Read the model definition and answer for the solid it produces. Units are mm, in the model's axes. A direction names the side the tool comes from. Give positions to 0.01 mm unless a question says otherwise; leave off trailing zeros. Write each loop counter-clockwise with the first axis right and the second up, starting at its lowest first coordinate (ties: lowest second). Pieces come first, ordered by that corner, then holes. Notation, with made-up numbers: (-19.75, 87.25) -> (31.25, 87.25) arc R15 cw to (31.25, 101.25) -> close; hole circle Ø6 at (13.5, 74). An arc over 180 degrees is marked (long way). Write item = value, one per line.
Autodesk Fusion 360 part; units mm, degrees
sketch "Sketch1" plane through (0, 0, 0) normal (0, 0, 1) x (1, 0, 0)
  line L0 (0, 0) -> (51, 0)
  line L1 (51, 0) -> (51, 144)
  line L2 (51, 144) -> (0, 144)
  line L3 (0, 144) -> (0, 0)
  line L4 (10, 10) -> (41, 10)
  line L5 (41, 10) -> (41, 134)
  line L6 (41, 134) -> (10, 134)
  line L7 (10, 134) -> (10, 10)
  dimension "d1" = 51
  dimension "d2" = 144
  dimension "d5" = 31
  dimension "d6" = 124
extrude "Extrude1" add sketch "Sketch1" along normal blind 13
sketch "Sketch2" plane through (0, 0, 0) normal (0, 0, -1) x (1, 0, 0)
  line L0 (10, -134) -> (10, -10)
  line L1 (10, -10) -> (41, -10)
  line L2 (41, -10) -> (41, -134)
  line L3 (41, -134) -> (10, -134)
  line L4 (0, 0) -> (0, -144)
  line L5 (0, -144) -> (51, -144)
  line L6 (51, -144) -> (51, 0)
  line L7 (51, 0) -> (0, 0)
  line L8 (41, -134) -> (10, -134)
  line L9 (10, -134) -> (10, -10)
  line L10 (10, -10) -> (41, -10)
  line L11 (41, -10) -> (41, -134)
extrude "Extrude2" add sketch "Sketch2" against normal blind 3 contours L0 L1 L2 L3 L8 L9 L10 L11
sketch "Sketch3" plane through (0, 0, 13) normal (0, 0, 1) x (-1, 0, 0)
  line L0 (-10, -10) -> (-10, -134)
  line L1 (-10, -134) -> (-41, -134)
  line L2 (-41, -134) -> (-41, -10)
  line L3 (-41, -10) -> (-10, -10)
  line L4 (0, -144) -> (0, 0)
  line L5 (0, 0) -> (-51, 0)
  line L6 (-51, 0) -> (-51, -144)
  line L7 (-51, -144) -> (0, -144)
  line L8 (-41, -48.7) -> (-41, -67.4)
  line L9 (-41, -48.7) -> (-51, -48.7)
  line L10 (-51, -48.7) -> (-51, -67.4)
  line L11 (-51, -67.4) -> (-41, -67.4)
  line L12 (-41, -67.4) -> (-41, -48.7)
  dimension "d11" = 38.7
  dimension "d12" = 18.7
  dimension "d13" = 18.7
extrude "Extrude3" cut sketch "Sketch3" against normal blind 10 contours L2 L6 L8 L9 L10 L11 L12
(1) The part is cut by section B-B on y = 47. Determine the outline of the cut face in (x, z).
Checks:
outline = (0, 0) -> (51, 0) -> (51, 13) -> (41, 13) -> (41, 3) -> (10, 3) -> (10, 13) -> (0, 13) -> close
(2) The part is cut by section A-A on x = 16. Determine the outline of the cut face in (y, z), plus the area to 3 significant figures.
Checks:
outline = (0, 0) -> (144, 0) -> (144, 13) -> (134, 13) -> (134, 3) -> (10, 3) -> (10, 13) -> (0, 13) -> close
area = 632 mm²
(3) Given P1, Ø5, axis at x = 45.5, z = 3.5, coming from the -Y side, flat-ended and moving along its own axis, determine where the tip first touches the part or whether it passes through.
Checks:
P1 = 0
(4) For a pull along X with two mould halves and no side action, classify faces 1 (the flat face through (26, 134, 8)), 2 (the flat face through (51, 71, 6)), 3 (the flat face through (46, 67.4, 8)) as released by +X, released by -X, zero draft, split by the parting line, or undercut.
Checks:
face_1 = undercut
face_2 = released by +X
face_3 = zero draft
(5) Consider L1, parallel to X at y = 15, z = 12.25; L2, parallel to Y at x = 38, z = 6.5; L3, parallel to Y at x = 43, z = 10.5. Determine where each line is inside the solid, lowest interval first.
Checks:
L1 = 0 to 10, 41 to 51
L2 = 0 to 10, 134 to 144
L3 = 0 to 48.7, 67.4 to 144
(6) A tool of negligible diameter and unlimited length cuts with its end or side. For faces 4 (the flat face through (8, 73, 13)), 5 (the flat face through (10, 73, 8)), 6 (the flat face through (46, 48.7, 8)), from which of +Z, -Z, +X, -X, +Y, -Y can it reach the whole face along a straight path? Write none if from no direction.
Checks:
face_4 = +Z, +X, -X, +Y, -Y
face_5 = +Z
face_6 = +Z, +X
(7) The part is cut by section C-C on z = 7. Determine the outline of the cut face in (x, y), plus the area to 3 significant figures.
Checks:
outline = (0, 0) -> (51, 0) -> (51, 48.7) -> (41, 48.7) -> (41, 10) -> (10, 10) -> (10, 134) -> (41, 134) -> (41, 67.4) -> (51, 67.4) -> (51, 144) -> (0, 144) -> close
area = 3,310 mm²
